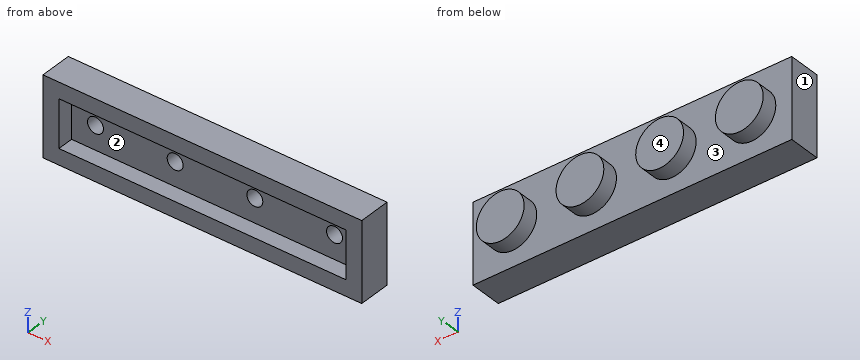
from build123d import *

# Parameters (mm, degrees)
SKETCH1_W           = 32
SKETCH1_H           = 8
BOSS_EXTRUDE1_DEPTH = 3.2
SKETCH2_R           = 2.4
BOSS_EXTRUDE2_DEPTH = 1.6
LPATTERN1_COUNT     = 4
LPATTERN1_PITCH     = 8
SHELL1_T            = -1.6


with BuildPart() as part:
    # Sketch1 → Boss-Extrude1 (new body)
    with BuildSketch(Plane(origin=(0, 0, 0), x_dir=(1, 0, 0), z_dir=(0, 1, 0))):
        with Locations((16, 4)):
            Rectangle(SKETCH1_W, SKETCH1_H)
    extrude(amount=BOSS_EXTRUDE1_DEPTH)

    # Sketch2 → Boss-Extrude2 (add)
    with BuildSketch(Plane(origin=(0, 3.2, 0), x_dir=(1, 0, 0), z_dir=(0, 1, 0))):
        with Locations(Location((28, 4, 0), (0, 0, 90))):
            Circle(SKETCH2_R)
    boss_extrude2 = extrude(amount=BOSS_EXTRUDE2_DEPTH)

    # LPattern1: Boss-Extrude2 ×4
    with Locations(*[(-i * LPATTERN1_PITCH, 0, 0) for i in range(1, LPATTERN1_COUNT)]):
        add(boss_extrude2)

    # Shell1
    shell1_openings = [part.faces().sort_by_distance(p)[0] for p in [
        (16, 0, -4),
    ]]
    offset(amount=SHELL1_T, openings=shell1_openings, kind=Kind.INTERSECTION)


solid = part.part
Work out the finished part from the listing and answer in its coordinate system (mm). Face numbers are marked on the shaded views. Round coordinates to 2 decimals unless told otherwise and drop trailing zeros. Write each loop counter-clockwise with the first axis right and the second up, starting at its lowest first coordinate (ties: lowest second). Pieces come first, ordered by that corner, then holes. Notation, with made-up numbers: (-2.5, 5.5) - (40.5, 5.5) arc R16 ccw to (40.5, 35.5) - close; hole circle Ø8 at (56, 11.5). An arc over 180 degrees is marked (long way). Answer in a Markdown table with one row per item. Add a question column.
1. A cutting plane is placed at A-A, the plane x = 15. Determine the outline of the cut face in (y, z), and give its area (3 significant figures).
2. Given pin 1 (1.8 mm diameter, centred on x = 4, z = -4, fed in from -Y); pin 2 (1.5 mm diameter, centred on x = 6.5, z = -2.5, fed in from +Y); pin 3 (1 mm diameter, centred on x = 20, z = -4, fed in from -Y), each flat-ended and moving along its own axis, determine where each tip first touches the part or whether it passes through.
3. A cutting plane is placed at B-B, the plane y = 4.35. Determine the outline of the cut face in (x, z).
4. A cutting plane is placed at D-D, the plane x = 20. Determine the outline of the cut face in (y, z).
5. The mould has two halves that part along X. Classify the marked faces 1, 2, 3 and 4: +X half, -X half, draft (parallel to the pull), parting line (faces both ways), or undercut.
6. Find the intervals of material crossed by line 1 along X through (y, z) = (2.5, -4); line 2 along Z through (x, y) = (15.5, 0.45); line 3 along X through (y, z) = (4.65, -2.5), in increasing order. Write a range as from..to.
7. A cutting plane is placed at C-C, the plane z = -5.5. Determine the outline of the cut face in (x, y).
Worked out:
| question | item | result |
|---|---|---|
| 1 | outline | (0, -8) - (3.2, -8) - (3.2, 0) - (0, 0) - (0, -1.6) - (1.6, -1.6) - (1.6, -6.4) - (0, -6.4) - close |
| 1 | area | 17.9 mm^2 |
| 2 | pin 1 | y = 1.6 |
| 2 | pin 2 | y = 4.8 |
| 2 | pin 3 | y = 3.2 |
| 3 | outline | circle Ø4.8 at (4, -4); circle Ø4.8 at (12, -4); circle Ø4.8 at (20, -4); circle Ø4.8 at (28, -4) |
| 4 | outline | (0, -8) - (3.2, -8) - (3.2, -6.4) - (4.8, -6.4) - (4.8, -1.6) - (3.2, -1.6) - (3.2, 0) - (0, 0) - (0, -1.6) - (1.6, -1.6) - (1.6, -3.2) - (3.2, -3.2) - (3.2, -4.8) - (1.6, -4.8) - (1.6, -6.4) - (0, -6.4) - close |
| 5 | face 1 | -X half |
| 5 | face 2 | undercut |
| 5 | face 3 | undercut |
| 5 | face 4 | draft |
| 6 | line 1 | 0..3.2, 4.8..11.2, 12.8..19.2, 20.8..27.2, 28.8..32 |
| 6 | line 2 | -8..-6.4, -1.6..0 |
| 6 | line 3 | 2.13..5.87, 10.13..13.87, 18.13..21.87, 26.13..29.87 |
| 7 | outline | (0, 0) - (1.6, 0) - (1.6, 1.6) - (30.4, 1.6) - (30.4, 0) - (32, 0) - (32, 3.2) - (29.87, 3.2) - (29.87, 4.8) - (26.13, 4.8) - (26.13, 3.2) - (21.87, 3.2) - (21.87, 4.8) - (18.13, 4.8) - (18.13, 3.2) - (13.87, 3.2) - (13.87, 4.8) - (10.13, 4.8) - (10.13, 3.2) - (5.87, 3.2) - (5.87, 4.8) - (2.13, 4.8) - (2.13, 3.2) - (0, 3.2) - close |
